Geometry: final body of the model. Coordinates: model frame, mm. Round coordinates to 2 decimals unless told otherwise and drop trailing zeros. Loops run counter-clockwise (first coordinate to the right, second up) from the corner with the lowest first, then second, coordinate; pieces in that order, holes last. Notation, with made-up numbers: M -1,-22 L 40,-22 A32 ccw 40,5 Z; hole C 40,45 d11. An arc over 180 degrees is marked long. Answer as a JSON object with one key per item and string values.
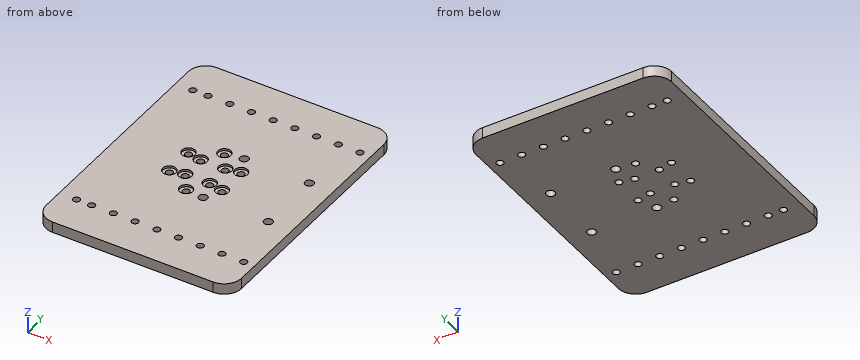
```python
from build123d import *

# Parameters (mm, degrees)
SKETCH_1_W            = 90
SKETCH_1_H            = 120
SKETCH_1_R            = 2
SKETCH_1_R_2          = 1.6
EXTRUDE_1_DEPTH       = 5
FILLET_1_R            = 8
F_3_2_PCD16_R         = 1.6
CUT_EXTRUDE_3_2_DEPTH = 10
XRU1008_6_1_2_R       = 3
XRU1008_6_1_DEPTH     = 1
XRU2012_3_2_28_2_R    = 1.6
XRU2012_3_2_28_DEPTH  = 5
XRU2012_6_1_2_R       = 3
XRU2012_6_1_DEPTH     = 1


with BuildPart() as part:
    # Sketch 1 → Extrude 1 (new body)
    with BuildSketch(Plane.XY):
        with Locations((45, -60)):
            Rectangle(SKETCH_1_W, SKETCH_1_H)
        with Locations((79, -45)):
            Circle(SKETCH_1_R, mode=Mode.SUBTRACT)
        with Locations((79, -75)):
            Circle(SKETCH_1_R, mode=Mode.SUBTRACT)
        with Locations((49, -45)):
            Circle(SKETCH_1_R, mode=Mode.SUBTRACT)
        with Locations((49, -75)):
            Circle(SKETCH_1_R, mode=Mode.SUBTRACT)
        with Locations((85, -102.5)):
            Circle(SKETCH_1_R_2, mode=Mode.SUBTRACT)
        with Locations((75, -102.5)):
            Circle(SKETCH_1_R_2, mode=Mode.SUBTRACT)
        with Locations((65, -102.5)):
            Circle(SKETCH_1_R_2, mode=Mode.SUBTRACT)
        with Locations((55, -102.5)):
            Circle(SKETCH_1_R_2, mode=Mode.SUBTRACT)
        with Locations((45, -102.5)):
            Circle(SKETCH_1_R_2, mode=Mode.SUBTRACT)
        with Locations((85, -17.5)):
            Circle(SKETCH_1_R_2, mode=Mode.SUBTRACT)
        with Locations((75, -17.5)):
            Circle(SKETCH_1_R_2, mode=Mode.SUBTRACT)
        with Locations((65, -17.5)):
            Circle(SKETCH_1_R_2, mode=Mode.SUBTRACT)
        with Locations((55, -17.5)):
            Circle(SKETCH_1_R_2, mode=Mode.SUBTRACT)
        with Locations((45, -17.5)):
            Circle(SKETCH_1_R_2, mode=Mode.SUBTRACT)
        with Locations((35, -102.5)):
            Circle(SKETCH_1_R_2, mode=Mode.SUBTRACT)
        with Locations((25, -102.5)):
            Circle(SKETCH_1_R_2, mode=Mode.SUBTRACT)
        with Locations((15, -102.5)):
            Circle(SKETCH_1_R_2, mode=Mode.SUBTRACT)
        with Locations((35, -17.5)):
            Circle(SKETCH_1_R_2, mode=Mode.SUBTRACT)
        with Locations((25, -17.5)):
            Circle(SKETCH_1_R_2, mode=Mode.SUBTRACT)
        with Locations((15, -17.5)):
            Circle(SKETCH_1_R_2, mode=Mode.SUBTRACT)
        with Locations((8, -102.5)):
            Circle(SKETCH_1_R_2, mode=Mode.SUBTRACT)
        with Locations((8, -17.5)):
            Circle(SKETCH_1_R_2, mode=Mode.SUBTRACT)
    extrude(amount=EXTRUDE_1_DEPTH)

    # Fillet 1
    fillet_1_edges = [part.edges().sort_by_distance(p)[0] for p in [
        (0, 0, 2.5),
        (90, 0, 2.5),
        (90, -120, 2.5),
        (0, -120, 2.5),
    ]]
    fillet(fillet_1_edges, radius=FILLET_1_R)

    # 3.2_PCD16 → Cut-Extrude 3.2 (cut)
    with BuildSketch(Plane(origin=(0, 0, 0), x_dir=(-1, 0, 0), z_dir=(0, 0, -1))):
        with Locations((-46.156854249, -54.343145751)):
            Circle(F_3_2_PCD16_R)
        with Locations((-34.843145751, -54.343145751)):
            Circle(F_3_2_PCD16_R)
        with Locations((-34.843145751, -65.656854249)):
            Circle(F_3_2_PCD16_R)
        with Locations((-46.156854249, -65.656854249)):
            Circle(F_3_2_PCD16_R)
    extrude(amount=-CUT_EXTRUDE_3_2_DEPTH, mode=Mode.SUBTRACT)

    # XRU1008__6___1 2 → XRU1008__6___1 (cut)
    with BuildSketch(Plane.XY.offset(5)):
        with Locations((46.156854249, -54.343145751)):
            Circle(XRU1008_6_1_2_R)
        with Locations((34.843145751, -54.343145751)):
            Circle(XRU1008_6_1_2_R)
        with Locations((34.843145751, -65.656854249)):
            Circle(XRU1008_6_1_2_R)
        with Locations((46.156854249, -65.656854249)):
            Circle(XRU1008_6_1_2_R)
    extrude(amount=-XRU1008_6_1_DEPTH, mode=Mode.SUBTRACT)

    # XRU2012__3.2___28 2 → XRU2012__3.2___28 (cut)
    with BuildSketch(Plane.XY.offset(5)):
        with Locations((52.624355653, -53)):
            Circle(XRU2012_3_2_28_2_R)
        with Locations((40.5, -46)):
            Circle(XRU2012_3_2_28_2_R)
        with Locations((28.375644347, -53)):
            Circle(XRU2012_3_2_28_2_R)
        with Locations((28.375644347, -67)):
            Circle(XRU2012_3_2_28_2_R)
        with Locations((40.5, -74)):
            Circle(XRU2012_3_2_28_2_R)
        with Locations((52.624355653, -67)):
            Circle(XRU2012_3_2_28_2_R)
    extrude(amount=-XRU2012_3_2_28_DEPTH, mode=Mode.SUBTRACT)

    # XRU2012__6___1 2 → XRU2012__6___1 (cut)
    with BuildSketch(Plane.XY.offset(5)):
        with Locations((52.624355653, -53)):
            Circle(XRU2012_6_1_2_R)
        with Locations((40.5, -46)):
            Circle(XRU2012_6_1_2_R)
        with Locations((28.375644347, -53)):
            Circle(XRU2012_6_1_2_R)
        with Locations((28.375644347, -67)):
            Circle(XRU2012_6_1_2_R)
        with Locations((40.5, -74)):
            Circle(XRU2012_6_1_2_R)
        with Locations((52.624355653, -67)):
            Circle(XRU2012_6_1_2_R)
    extrude(amount=-XRU2012_6_1_DEPTH, mode=Mode.SUBTRACT)


solid = part.part
```
1) Line query: probe 1 along Y at (x, z) = (79, 2.55); probe 2 along Y at (x, z) = (26, 1.65); probe 3 along X at (y, z) = (-53.5, 0.4). Output: solid intervals per line, ascending.
Geometry results:
{"probe 1": "-120 to -77, -73 to -47, -43 to 0", "probe 2": "-120 to -103.75, -101.25 to -18.75, -16.25 to 0", "probe 3": "0 to 26.86, 29.9 to 33.48, 36.2 to 44.8, 47.52 to 51.1, 54.14 to 90"}
2) Cut plane B-B on y = -17.5. Count the separate pieces of the cut face and the enclosed holes in it, and give its area (3 significant figures).
Geometry results:
{"separate pieces": "10", "enclosed holes": "0", "area": "306 mm2"}
3) First-contact query: pin 1 (3.5 mm diameter, centred on x = 40.5, y = -46, fed in from -Z); pin 2 (5 mm diameter, centred on x = 52.62, y = -53, fed in from +Z). Flat tips, straight axial feed; report the tip coordinate or a pass-through.
Geometry results:
{"pin 1": "z = 0", "pin 2": "z = 4"}
4) Cut plane A-A on x = 40.5. Return the cut outline in (y, z), and give its area (3 significant figures).
Geometry results:
{"outline": "M -120,0 L -75.6,0 L -75.6,4 L -77,4 L -77,5 L -120,5 Z; M -72.4,0 L -47.6,0 L -47.6,4 L -49,4 L -49,5 L -71,5 L -71,4 L -72.4,4 Z; M -44.4,0 L 0,0 L 0,5 L -43,5 L -43,4 L -44.4,4 Z", "area": "562 mm2"}
5) Cut plane C-C on x = 79. Return the cut outline in (y, z), and give its area (3 significant figures).
Geometry results:
{"outline": "M -120,0 L -77,0 L -77,5 L -120,5 Z; M -73,0 L -47,0 L -47,5 L -73,5 Z; M -43,0 L 0,0 L 0,5 L -43,5 Z", "area": "560 mm2"}
